from build123d import *

# Parameters (mm, degrees)
SKETCH1_R           = 1.905
SKETCH1_R_2         = 1.27
BOSS_EXTRUDE1_DEPTH = 3.175
SKETCH2_R           = 1.27
CUT_EXTRUDE1_DEPTH  = 3.175
FILLET1_R           = 6.35
SKETCH3_W           = 9.525
SKETCH3_H           = 9.525
BOSS_EXTRUDE2_DEPTH = 3.175
FILLET2_R           = 1.5875


with BuildPart() as part:
    # Sketch1 → Boss-Extrude1 (new body)
    with BuildSketch(Plane(origin=(0, 0, 0), x_dir=(1, 0, 0), z_dir=(0, 1, 0))):
        Polygon((-82.55, 31.75), (-82.55, -44.45), (44.45, -44.45), (44.45, 4.889379277), (-57.15, 31.75), align=None)
        Circle(SKETCH1_R, mode=Mode.SUBTRACT)
        with Locations((-57.15, 25.774227063)):
            Circle(SKETCH1_R_2, mode=Mode.SUBTRACT)
        with Locations((-76.2, 25.4)):
            Circle(SKETCH1_R, mode=Mode.SUBTRACT)
        with Locations((38.1, 0)):
            Circle(SKETCH1_R, mode=Mode.SUBTRACT)
    extrude(amount=BOSS_EXTRUDE1_DEPTH)

    # Sketch2 → Cut-Extrude1 (cut)
    with BuildSketch(Plane(origin=(0, 3.175, 0), x_dir=(1, 0, 0), z_dir=(0, 1, 0))):
        with Locations((-76.2, 12.192)):
            Circle(SKETCH2_R)
        with Locations((-10.922, 12.192)):
            Circle(SKETCH2_R)
        with Locations((-10.922, -31.75)):
            Circle(SKETCH2_R)
        with Locations((-76.2, -31.75)):
            Circle(SKETCH2_R)
        with BuildLine():
            Line((-69.85, 10.16), (-69.85, -26.035))
            ThreePointArc((-69.85, -26.035), (-69.106051224, -27.831051224), (-67.31, -28.575))
            Line((-67.31, -28.575), (-8.89, -28.575))
            ThreePointArc((-8.89, -28.575), (-7.093948776, -27.831051224), (-6.35, -26.035))
            Line((-6.35, -26.035), (-6.35, -19.674755399))
            ThreePointArc((-6.35, -19.674755399), (-6.755973152, -18.297246992), (-7.844117647, -17.360078293))
            ThreePointArc((-7.844117647, -17.360078293), (-18.033037532, -6.14101436), (-16.808823529, 8.964705882))
            ThreePointArc((-16.808823529, 8.964705882), (-16.871967969, 11.466819219), (-19.05, 12.7))
            Line((-19.05, 12.7), (-67.31, 12.7))
            ThreePointArc((-67.31, 12.7), (-69.106051224, 11.956051224), (-69.85, 10.16))
        make_face()
        with BuildLine():
            Line((6.35, -19.674755399), (6.35, -26.035))
            ThreePointArc((6.35, -26.035), (7.093948776, -27.831051224), (8.89, -28.575))
            Line((8.89, -28.575), (29.21, -28.575))
            ThreePointArc((29.21, -28.575), (31.006051224, -27.831051224), (31.75, -26.035))
            Line((31.75, -26.035), (31.75, -6.845130987))
            ThreePointArc((31.75, -6.845130987), (31.222535045, -5.295517264), (29.859210479, -4.38949955))
            Line((29.859210479, -4.38949955), (21.722749497, -2.23841301))
            ThreePointArc((21.722749497, -2.23841301), (19.753320798, -2.524108077), (18.594299133, -4.141803924))
            ThreePointArc((18.594299133, -4.141803924), (14.779315437, -12.019747718), (7.844117647, -17.360078293))
            ThreePointArc((7.844117647, -17.360078293), (6.755973152, -18.297246992), (6.35, -19.674755399))
        make_face()
    extrude(amount=-CUT_EXTRUDE1_DEPTH, mode=Mode.SUBTRACT)

    # Fillet1
    fillet1_edges = [part.edges().sort_by_distance(p)[0] for p in [
        (-57.15, 1.5875, -31.75),
        (44.45, 1.5875, -4.889379277),
        (-82.55, 1.5875, -31.75),
    ]]
    fillet(fillet1_edges, radius=FILLET1_R)

    # Sketch3 → Boss-Extrude2 (add)
    with BuildSketch(Plane.XY.offset(44.45)):
        with Locations((-77.7875, 7.9375)):
            Rectangle(SKETCH3_W, SKETCH3_H)
        Polygon((-77.7875, 5.243423164), (-75.093423164, 7.9375), (-77.7875, 10.631576836), (-80.481576836, 7.9375), align=None, mode=Mode.SUBTRACT)
        with Locations((39.6875, 7.9375)):
            Rectangle(SKETCH3_W, SKETCH3_H)
        Polygon((39.6875, 5.243423164), (42.381576836, 7.9375), (39.6875, 10.631576836), (36.993423164, 7.9375), align=None, mode=Mode.SUBTRACT)
        with Locations((-19.05, 7.9375)):
            Rectangle(SKETCH3_W, SKETCH3_H)
        Polygon((-19.05, 5.243423164), (-16.355923164, 7.9375), (-19.05, 10.631576836), (-21.744076836, 7.9375), align=None, mode=Mode.SUBTRACT)
    extrude(amount=-BOSS_EXTRUDE2_DEPTH)

    # Fillet2
    fillet2_edges = [part.edges().sort_by_distance(p)[0] for p in [
        (-82.55, 12.7, 42.8625),
        (-73.025, 12.7, 42.8625),
        (-77.7875, 3.175, 41.275),
        (-73.025, 3.175, 42.8625),
        (44.45, 12.7, 42.8625),
        (39.6875, 3.175, 41.275),
        (34.925, 3.175, 42.8625),
        (34.925, 12.7, 42.8625),
        (-23.8125, 3.175, 42.8625),
        (-23.8125, 12.7, 42.8625),
        (-14.2875, 12.7, 42.8625),
        (-19.05, 3.175, 41.275),
        (-14.2875, 3.175, 42.8625),
    ]]
    fillet(fillet2_edges, radius=FILLET2_R)


solid = part.part
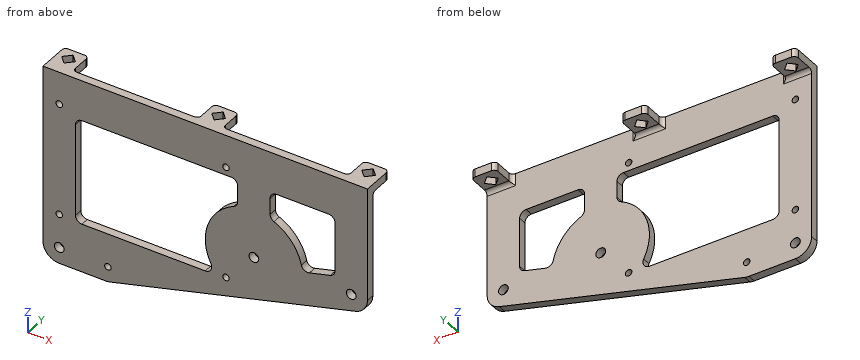
The listing builds one solid part. Answer for the finished solid, in the listing's coordinates (mm). Coordinates: 2 decimals unless noted, no trailing zeros. Loops run counter-clockwise (first coordinate to the right, second up) from the corner with the lowest first, then second, coordinate; pieces in that order, holes last.
1) Find the intervals of material crossed by L1, parallel to Z at x = -76.2, y = 1.9 (3 decimals); L2, parallel to X at y = 0.8, z = 0 (3 decimals); L3, parallel to Z at x = -26, y = 2.5 (3 decimals), in increasing order.
2) Flat-ended cylindrical pins translate along their axes: pin 1 Ø6 at (x, y) = (-34, 3.5) entering from -Z; pin 2 Ø2.5 at (x, z) = (0, 0) entering from -Y; pin 3 Ø2.5 at (x, y) = (38, 8) entering from -Z (3 decimals); pin 4 Ø4 at (x, z) = (-4, 16.5) entering from +Y (3 decimals). Find the tip coordinate at first contact, or state that the pin passes through.
3) Find section D-D on x = -27. Write down the section's boundary in (y, z) (3 decimals), then the cut area to 3 significant figures.
4) Find section A-A on z = 31.75. Write down the section's boundary in (x, y) (3 decimals), then the cut area to 3 significant figures.
5) Find section C-C on y = 9.25. Give the number of separate pieces and of enclosed holes in the cut face, then the cut area to 3 significant figures.
6) Find section B-B on x = 0. Write down the section's boundary in (y, z) (3 decimals).
Values:
1. L1: z = -31.75 to -27.305, -23.495 to -13.462, -10.922 to 30.48, 33.02 to 44.45
1. L2: x = -82.55 to -69.85, -19.05 to -1.905, 1.905 to 36.195, 40.005 to 44.45
1. L3: z = -23.515 to -12.7, 28.575 to 44.45
2. pin 1: stops at z = -26.42
2. pin 2: passes through
2. pin 3: stops at z = 41.275
2. pin 4: stops at y = 3.175
3. outline: (0, -23.779) - (3.175, -23.779) - (3.175, -12.7) - (0, -12.7) - close; (0, 28.575) - (3.175, 28.575) - (3.175, 44.45) - (0, 44.45) - close
3. area: 85.6 mm2
4. outline: (-82.55, 0) - (-77.47, 0) - (-77.47, 3.175) - (-82.55, 3.175) - close; (-74.93, 0) - (-12.192, 0) - (-12.192, 3.175) - (-74.93, 3.175) - close; (-9.652, 0) - (44.45, 0) - (44.45, 3.175) - (-9.652, 3.175) - close
4. area: 387 mm2
5. separate pieces: 6
5. enclosed holes: 0
5. area: 64.4 mm2
6. outline: (0, -16.641) - (3.175, -16.641) - (3.175, -1.905) - (0, -1.905) - close; (0, 1.905) - (3.175, 1.905) - (3.175, 44.45) - (0, 44.45) - close
